For this review, take the finished solid that the model builds, in its own axes (mm). A direction names the side the tool comes from. Round coordinates to 2 decimals unless told otherwise and drop trailing zeros. Order: outer loops, then holes, each group sorted by start corner. A loop starts at its lowest first (then second) coordinate and runs counter-clockwise, first axis right, second up. Notation, with made-up numbers: M -4.5,45 L 4.5,45 A27 cw 4.5,70 Z; hole C 19,-7 d2. An arc over 180 degrees is marked long. Write item = value, one per line. Start each with the question number.
from build123d import *

# Parameters (mm, degrees)
EXTRUDE_1_DEPTH     = 15
SKETCH_2_R          = 1.6
CUT_EXTRUDE_1_DEPTH = 25
CUT_EXTRUDE_2_DEPTH = 25
RIB_1_REACH         = 37.355
SKETCH_4_WALL_W     = 93.3019384
SKETCH_4_WALL_H     = 5
FILLET_1_R          = 2


with BuildPart() as part:
    # 草图1 → 凸台-拉伸1 (new, symmetric)
    with BuildSketch(Plane.XY):
        Polygon((0, 0), (0, 25), (-3, 25), (-3, -3), (20, -3), (20, 0), align=None)
    extrude(amount=EXTRUDE_1_DEPTH, both=True)

    # 草图2 → 切除-拉伸1 (cut)
    with BuildSketch(Plane(origin=(0, 0, 0), x_dir=(1, 0, 0), z_dir=(0, 1, 0))):
        with Locations(Location((10, -8, 0), (0, 0, 180))):
            Circle(SKETCH_2_R)
        with Locations(Location((10, 8, 0), (0, 0, 180))):
            Circle(SKETCH_2_R)
    extrude(amount=-CUT_EXTRUDE_1_DEPTH, mode=Mode.SUBTRACT)

    # 草图3 → 切除-拉伸2 (cut)
    with BuildSketch(Plane.ZY.offset(3)):
        with BuildLine():
            Line((-11.5, 21.25), (-8.5, 21.25))
            ThreePointArc((-8.5, 21.25), (-7.25, 20), (-8.5, 18.75))
            Line((-8.5, 18.75), (-11.5, 18.75))
            ThreePointArc((-11.5, 18.75), (-12.75, 20), (-11.5, 21.25))
        make_face()
        with BuildLine():
            Line((11.5, 21.25), (8.5, 21.25))
            ThreePointArc((8.5, 21.25), (7.25, 20), (8.5, 18.75))
            Line((8.5, 18.75), (11.5, 18.75))
            ThreePointArc((11.5, 18.75), (12.75, 20), (11.5, 21.25))
        make_face()
    extrude(amount=-CUT_EXTRUDE_2_DEPTH, mode=Mode.SUBTRACT)

    # 草图4 wall → 筋1 (add, up to next)
    with BuildSketch(Plane(origin=(5, 9, 0), x_dir=(0.485642931179, -0.874157276122, 0), z_dir=(0.874157276122, 0.485642931179, 0)), mode=Mode.PRIVATE) as rib_1_sk1:
        Rectangle(SKETCH_4_WALL_W, SKETCH_4_WALL_H)
    rib_1_tool1 = extrude(rib_1_sk1.sketch, amount=-RIB_1_REACH, mode=Mode.PRIVATE) - part.part
    add(rib_1_tool1.solids().sort_by_distance((5, 9, 0))[0])

    # 圆角1
    fillet_1_edges = [part.edges().sort_by_distance(p)[0] for p in [
        (0, 0, 8.75),
        (-1.5, 25, 15),
        (20, -1.5, 15),
        (20, -1.5, -15),
        (0, 0, -8.75),
        (10, 0, 0),
        (-1.5, 25, -15),
        (0, 18, 0),
    ]]
    fillet(fillet_1_edges, radius=FILLET_1_R)


solid = part.part
(1) For faces 1 (the flat face through (5, 9, 0)), 2 (the cylindrical face through (0.57, 0.6, 8.66)), 3 (the cylindrical face through (-1.52, 20.03, 7.25)), 4 (the flat face through (4, 6, -2.5)), 5 (the flat face through (0, 13, 4)), list the 3-axis set-ups (+Z, -Z, +X, -X, +Y, -Y) from which the entire face can be reached by the end or side of a thin tool; tool diameter is ignored.
(2) We need section C-C, the plane x = 5.5. Write out the cut boundary in (y, z).
(3) For line 1 along Z through (x, y) = (10, -1.6); line 2 along X through (y, z) = (22, 7), list the stretches that pass through material, from the lowest coordinate up.
(4) We need section D-D, the plane z = -8. Write out the cut boundary in (x, y).
(5) We need section A-A, the plane y = 20. Write out the cut boundary in (x, z).
(6) Draft analysis for pull direction Y (two halves, no side actions). For faces 6 (the flat face through (-2, 18.75, -10)), 7 (the flat face through (4, 6, 2.5)), 8 (the flat face through (8, -3, 0)), 9 (the cylindrical face through (0.062, 18.023, -0.035)), state which applies: released by +Y, released by -Y, zero draft, split by the parting line, or undercut.
(7) Insertion check: pin 1 (1 mm diameter, centred on y = 14, z = 4, fed in from +X); pin 2 (12.5 mm diameter, centred on x = 6.5, y = 10.5, fed in from +Z); pin 3 (3 mm diameter, centred on x = 16, z = 0, fed in from +Y). Each pin has a flat end and moves straight along its axis. Give the tip position at first contact, or say it passes through.
(8) We need section B-B, the plane z = 4.75. Write out the cut boundary in (x, y), then the cut area to 3 significant figures.
Values:
q1.face_1 = +Z, -Z, +X, +Y
q1.face_2 = +Z, +X, +Y
q1.face_3 = +X, -X
q1.face_4 = -Z, +X, +Y
q1.face_5 = +X, +Y
q2.outline = M -3,-15 L 0,-15 L 0,-2.5 L 8.1,-2.5 L 8.1,2.5 L 0,2.5 L 0,15 L -3,15 Z
q3.line_1 = -15 to -9.6, -6.4 to 6.4, 9.6 to 15
q3.line_2 = -3 to 0
q4.outline = M -3,-3 L 8.4,-3 L 8.4,0 L 2,0 A2 cw 0,2 L 0,18.85 L -3,18.85 Z; M -3,21.15 L 0,21.15 L 0,25 L -3,25 Z; M 11.6,-3 L 20,-3 L 20,0 L 11.6,0 Z
q5.outline = M -3,-15 L 0,-15 L 0,-12.75 L -3,-12.75 Z; M -3,-7.25 L 0,-7.25 L 0,7.25 L -3,7.25 Z; M -3,12.75 L 0,12.75 L 0,15 L -3,15 Z
q6.face_6 = undercut
q6.face_7 = zero draft
q6.face_8 = released by -Y
q6.face_9 = released by +Y
q7.pin_1 = 0
q7.pin_2 = 2.5
q7.pin_3 = 0
q8.outline = M -3,-3 L 20,-3 L 20,0 L 2,0 A2 cw 0,2 L 0,25 L -3,25 Z
q8.area = 145 mm²
